The listing builds one solid part. Answer for the finished solid, in the listing's coordinates (mm). Face numbers are marked on the shaded views. A direction names the side the tool comes from. Round coordinates to 2 decimals unless told otherwise and drop trailing zeros. Write each loop counter-clockwise with the first axis right and the second up, starting at its lowest first coordinate (ties: lowest second). Pieces come first, ordered by that corner, then holes. Notation, with made-up numbers: (46, 17) - (51, 17) arc R30 ccw to (51, 56) - close; hole circle Ø1 at (-1, -21). An arc over 180 degrees is marked (long way). Use a Markdown table: item, result. Add a question column.
1) Each of these flat-tipped pins is pushed along its axis until it touches: P1, Ø5.5, axis at x = 1, z = 5.5, coming from the +Y side; P2, Ø6, axis at x = -1, y = 45, coming from the -Z side; P3, Ø4, axis at x = 0, y = 50.8, coming from the -Z side; P4, Ø4, axis at x = -1, y = 31.5, coming from the +Z side. Where does it stop, or does it pass through?
2) A cutting plane is placed at B-B (z = 13). Give the vertices of the cut face in (x, y), then the cut area to 4 significant figures.
3) A cutting plane is placed at D-D (y = -1). Give the vertices of the cut face in (x, z), then the cut area to 3 significant figures.
4) Determine the mould class of the marked faces 1, 2, 3 and 4 for opening direction X: +X half, -X half, draft (parallel to the pull), parting line (faces both ways), or undercut.
5) A cutting plane is placed at C-C (x = 1). Give the vertices of the cut face in (y, z), then the cut area to 3 significant figures.
6) A cutting plane is placed at A-A (y = 26.5). Give the vertices of the cut face in (x, z), then the cut area to 3 significant figures.
7) A tool of negligible diameter and unlimited length cuts with its end or side. For the marked faces 5, 6, 7, 8 and 9, from which of +Z, -Z, +X, -X, +Y, -Y can it reach the whole face along a straight path? Write none if from no direction.
8) Find the intervals of material crossed by probe 1 along Y at (x, z) = (0, 1.35) (3 decimals); probe 2 along Z at (x, y) = (-3, -3); probe 3 along Y at (x, z) = (1.75, 1), in increasing order. Write a range as from..to.
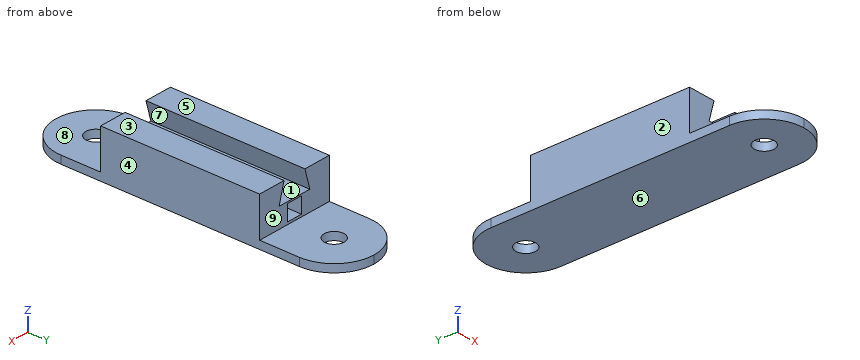
```python
from build123d import *

# Parameters (mm, degrees)
SKETCH1_W           = 25.4
SKETCH1_H           = 25.4
SKETCH1_R           = 3.175
SKETCH1_H_2         = 50.8
BOSS_EXTRUDE1_DEPTH = 2.54
SKETCH1_3_W         = 25.4
SKETCH1_3_H         = 50.8
BOSS_EXTRUDE2_DEPTH = 15.24
CUT_EXTRUDE1_DEPTH  = 79.74
FILLET1_R           = 12.7
SKETCH4_W           = 5.08
SKETCH4_H           = 5.08
CUT_EXTRUDE2_DEPTH  = 20.32


with BuildPart() as part:
    # Sketch1 → Boss-Extrude1 (new body)
    # profile 1 of 3: a face of its own
    with BuildSketch(Plane.XY):
        with Locations((0, 50.8)):
            Rectangle(SKETCH1_W, SKETCH1_H)
        with Locations((0, 50.8)):
            Circle(SKETCH1_R, mode=Mode.SUBTRACT)
    # profile 2 of 3: a face of its own
    with BuildSketch(Plane.XY):
        with Locations((0, 12.7)):
            Rectangle(SKETCH1_W, SKETCH1_H_2)
    # profile 3 of 3: a face of its own
    with BuildSketch(Plane.XY):
        with Locations((0, -25.4)):
            Rectangle(SKETCH1_W, SKETCH1_H)
        with Locations((0, -25.4)):
            Circle(SKETCH1_R, mode=Mode.SUBTRACT)
    extrude(amount=BOSS_EXTRUDE1_DEPTH)

    # Sketch1<3> → Boss-Extrude2 (add)
    with BuildSketch(Plane.XY):
        with Locations((0, 12.7)):
            Rectangle(SKETCH1_3_W, SKETCH1_3_H)
    extrude(amount=BOSS_EXTRUDE2_DEPTH)

    # Sketch3 → Cut-Extrude1 (cut, through all)
    with BuildSketch(Plane(origin=(0, 38.1, 0), x_dir=(1, 0, 0), z_dir=(0, 1, 0))):
        Polygon((-5.588, -8.89), (-3.81, -15.24), (3.81, -15.24), (5.588, -8.89), align=None)
    extrude(amount=-CUT_EXTRUDE1_DEPTH, mode=Mode.SUBTRACT)

    # Fillet1
    fillet1_edges = [part.edges().sort_by_distance(p)[0] for p in [
        (12.7, -38.1, 1.27),
        (-12.7, -38.1, 1.27),
        (12.7, 63.5, 1.27),
        (-12.7, 63.5, 1.27),
    ]]
    fillet(fillet1_edges, radius=FILLET1_R - 0.0001)  # a hair under: the kernel refuses the full size

    # Sketch4 → Cut-Extrude2 (cut)
    with BuildSketch(Plane(origin=(0, 38.1, 0), x_dir=(1, 0, 0), z_dir=(0, 1, 0))):
        with Locations((0, -5.842)):
            Rectangle(SKETCH4_W, SKETCH4_H)
    extrude(amount=-CUT_EXTRUDE2_DEPTH, mode=Mode.SUBTRACT)


solid = part.part
```
Entries:
| question | item | result |
|---|---|---|
| 1 | P1 | stops at y = 38.1 |
| 1 | P2 | stops at z = 0 |
| 1 | P3 | passes through |
| 1 | P4 | stops at z = 8.89 |
| 2 | outline | (-12.7, -12.7) - (-4.44, -12.7) - (-4.44, 38.1) - (-12.7, 38.1) - close; (4.44, -12.7) - (12.7, -12.7) - (12.7, 38.1) - (4.44, 38.1) - close |
| 2 | area | 839.5 mm² |
| 3 | outline | (-12.7, 0) - (12.7, 0) - (12.7, 15.24) - (3.81, 15.24) - (5.59, 8.89) - (-5.59, 8.89) - (-3.81, 15.24) - (-12.7, 15.24) - close |
| 3 | area | 327 mm² |
| 4 | face 1 | undercut |
| 4 | face 2 | -X half |
| 4 | face 3 | draft |
| 4 | face 4 | +X half |
| 5 | outline | (-38.06, 0) - (-28.41, 0) - (-28.41, 2.54) - (-38.06, 2.54) - close; (-22.39, 0) - (47.79, 0) - (47.79, 2.54) - (38.1, 2.54) - (38.1, 3.3) - (17.78, 3.3) - (17.78, 8.38) - (38.1, 8.38) - (38.1, 8.89) - (-12.7, 8.89) - (-12.7, 2.54) - (-22.39, 2.54) - close; (53.81, 0) - (63.46, 0) - (63.46, 2.54) - (53.81, 2.54) - close |
| 5 | area | 447 mm² |
| 6 | outline | (-12.7, 0) - (12.7, 0) - (12.7, 15.24) - (3.81, 15.24) - (5.59, 8.89) - (-5.59, 8.89) - (-3.81, 15.24) - (-12.7, 15.24) - close; hole (-2.54, 3.3) - (2.54, 3.3) - (2.54, 8.38) - (-2.54, 8.38) - close |
| 6 | area | 302 mm² |
| 7 | face 5 | +Z, +X, -X, +Y, -Y |
| 7 | face 6 | -Z, +X, -X, +Y, -Y |
| 7 | face 7 | +Y, -Y |
| 7 | face 8 | +Z, +X, -X, -Y |
| 7 | face 9 | +Z, +X, -X, +Y |
| 8 | probe 1 | y = -38.1..-28.575, -22.225..47.625, 53.975..63.5 |
| 8 | probe 2 | z = 0..8.89 |
| 8 | probe 3 | y = -37.98..-28.05, -22.75..48.15, 53.45..63.38 |
